CAD build for the part. Positions are in the model's coordinates, mm. Face numbers are marked on the shaded views. Coordinates: 2 decimals unless noted, no trailing zeros. Order: outer loops, then holes, each group sorted by start corner. A loop starts at its lowest first (then second) coordinate and runs counter-clockwise, first axis right, second up. Notation, with made-up numbers: M 68.25,13 L 83.25,13 A21 ccw 83.25,51 Z; hole C -16,38 d11. An arc over 180 degrees is marked long. One line per item, written item: value.
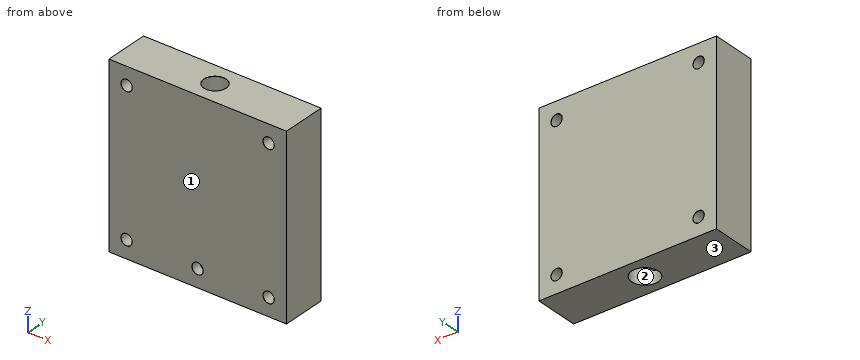
from build123d import *

# Parameters (mm, degrees)
ESQUISSE1_W                                         = 40
ESQUISSE1_H                                         = 40
BOSS_EXTRU_1_DEPTH                                  = 10
DIAM_TRE_DU_PER_AGE_4_0_4_1_D                       = 4
TROU_POUR_TARAUDAGE_POUR_TROU_TARAUD_M6_D           = 5
TROU_POUR_TARAUDAGE_POUR_TROU_TARAUD_M6_DEPTH       = 8
TROU_POUR_TARAUDAGE_POUR_TROU_TARAUD_M6_CSINK_D     = 5.05
TROU_POUR_TARAUDAGE_POUR_TROU_TARAUD_M6_CSINK_ANGLE = 90
TROU_POUR_TARAUDAGE_POUR_TROU_TARAUD_M6_TIP         = 1.502151548
DIAM_TRE_DU_PER_AGE_6_0_6_1_D                       = 6
DIAM_TRE_DU_PER_AGE_6_0_6_1_DEPTH                   = 20
DIAM_TRE_DU_PER_AGE_6_0_6_1_TIP                     = 1.802581857
TROU_POUR_TARAUDAGE_POUR_TROU_TARAUD_2_COUNT        = 2
TROU_POUR_TARAUDAGE_POUR_TROU_TARAUD_2_PITCH        = 32
TROU_POUR_TARAUDAGE_POUR_TROU_TARAUD_3_COUNT        = 2
TROU_POUR_TARAUDAGE_POUR_TROU_TARAUD_3_PITCH        = 45.254833996
TROU_POUR_TARAUDAGE_POUR_TROU_TARAUD_4_COUNT        = 2
TROU_POUR_TARAUDAGE_POUR_TROU_TARAUD_4_PITCH        = 32
TROU_POUR_TARAUDAGE_POUR_TROU_TARAUD_5_D            = 2.5
TROU_POUR_TARAUDAGE_POUR_TROU_TARAUD_5_DEPTH        = 5
TROU_POUR_TARAUDAGE_POUR_TROU_TARAUD_5_CSINK_D      = 2.55
TROU_POUR_TARAUDAGE_POUR_TROU_TARAUD_5_CSINK_ANGLE  = 90
TROU_POUR_TARAUDAGE_POUR_TROU_TARAUD_5_TIP          = 0.751075774


with BuildPart() as part:
    # Esquisse1 → Boss.-Extru.1 (new body)
    with BuildSketch(Plane(origin=(0, 0, 0), x_dir=(1, 0, 0), z_dir=(0, 1, 0))):
        with Locations((20, 20)):
            Rectangle(ESQUISSE1_W, ESQUISSE1_H)
    extrude(amount=BOSS_EXTRU_1_DEPTH)

    # Diamètre du perçage Ø4.0 (4)1 (through all)
    with Locations(Plane.XY):
        with Locations((20, 5)):
            Hole(DIAM_TRE_DU_PER_AGE_4_0_4_1_D / 2)

    # Trou pour taraudage pour trou taraudé M61
    with Locations(Plane.XY):
        with Locations((20, 5)):
            CounterSinkHole(TROU_POUR_TARAUDAGE_POUR_TROU_TARAUD_M6_D / 2, TROU_POUR_TARAUDAGE_POUR_TROU_TARAUD_M6_CSINK_D / 2, depth=TROU_POUR_TARAUDAGE_POUR_TROU_TARAUD_M6_DEPTH, counter_sink_angle=TROU_POUR_TARAUDAGE_POUR_TROU_TARAUD_M6_CSINK_ANGLE)
            with Locations((0, 0, -(TROU_POUR_TARAUDAGE_POUR_TROU_TARAUD_M6_DEPTH + TROU_POUR_TARAUDAGE_POUR_TROU_TARAUD_M6_TIP / 2))):  # 118° drill point
                Cone(0, TROU_POUR_TARAUDAGE_POUR_TROU_TARAUD_M6_D / 2, TROU_POUR_TARAUDAGE_POUR_TROU_TARAUD_M6_TIP, mode=Mode.SUBTRACT)

    # Diamètre du perçage Ø6.0 (6)1
    with Locations(Plane(origin=(0, 0, -40), x_dir=(-1, 0, 0), z_dir=(0, 0, -1))):
        with Locations((-20, 5)):
            Hole(DIAM_TRE_DU_PER_AGE_6_0_6_1_D / 2, depth=DIAM_TRE_DU_PER_AGE_6_0_6_1_DEPTH)
            with Locations((0, 0, -(DIAM_TRE_DU_PER_AGE_6_0_6_1_DEPTH + DIAM_TRE_DU_PER_AGE_6_0_6_1_TIP / 2))):  # 118° drill point
                Cone(0, DIAM_TRE_DU_PER_AGE_6_0_6_1_D / 2, DIAM_TRE_DU_PER_AGE_6_0_6_1_TIP, mode=Mode.SUBTRACT)

    # Esquisse17 → Trou pour taraudage pour trou taraud_ M3 (revolve, cut)
    with BuildSketch(Plane(origin=(4, 0, -4), x_dir=(0, 0, -1), z_dir=(1, 0, 0))):
        Polygon((0, 0), (0, 10), (1.275, 10), (1.25, 9.975), (1.25, 0.025), (1.275, 0), align=None)
    trou_pour_taraudage_pour_trou_taraud_m3 = revolve(axis=Axis((4, -6.35, -4), (0, 1, 0)), mode=Mode.SUBTRACT)

    # Trou pour taraudage pour trou taraud 2: Trou pour taraudage pour trou taraud_ M3 ×2
    with Locations(*[(i * TROU_POUR_TARAUDAGE_POUR_TROU_TARAUD_2_PITCH, 0, 0) for i in range(1, TROU_POUR_TARAUDAGE_POUR_TROU_TARAUD_2_COUNT)]):
        add(trou_pour_taraudage_pour_trou_taraud_m3, mode=Mode.SUBTRACT)

    # Trou pour taraudage pour trou taraud 3: Trou pour taraudage pour trou taraud_ M3 ×2
    with Locations(*[Vector(0.7071067811865475, 0, -0.7071067811865476) * (i * TROU_POUR_TARAUDAGE_POUR_TROU_TARAUD_3_PITCH) for i in range(1, TROU_POUR_TARAUDAGE_POUR_TROU_TARAUD_3_COUNT)]):
        add(trou_pour_taraudage_pour_trou_taraud_m3, mode=Mode.SUBTRACT)

    # Trou pour taraudage pour trou taraud 4: Trou pour taraudage pour trou taraud_ M3 ×2
    with Locations(*[(0, 0, -i * TROU_POUR_TARAUDAGE_POUR_TROU_TARAUD_4_PITCH) for i in range(1, TROU_POUR_TARAUDAGE_POUR_TROU_TARAUD_4_COUNT)]):
        add(trou_pour_taraudage_pour_trou_taraud_m3, mode=Mode.SUBTRACT)

    # Trou pour taraudage pour trou taraud 5
    with Locations(Plane(origin=(0, 0, 0), x_dir=(-1, 0, 0), z_dir=(0, -1, 0))):
        with Locations((-20, 36)):
            CounterSinkHole(TROU_POUR_TARAUDAGE_POUR_TROU_TARAUD_5_D / 2, TROU_POUR_TARAUDAGE_POUR_TROU_TARAUD_5_CSINK_D / 2, depth=TROU_POUR_TARAUDAGE_POUR_TROU_TARAUD_5_DEPTH, counter_sink_angle=TROU_POUR_TARAUDAGE_POUR_TROU_TARAUD_5_CSINK_ANGLE)
            with Locations((0, 0, -(TROU_POUR_TARAUDAGE_POUR_TROU_TARAUD_5_DEPTH + TROU_POUR_TARAUDAGE_POUR_TROU_TARAUD_5_TIP / 2))):  # 118° drill point
                Cone(0, TROU_POUR_TARAUDAGE_POUR_TROU_TARAUD_5_D / 2, TROU_POUR_TARAUDAGE_POUR_TROU_TARAUD_5_TIP, mode=Mode.SUBTRACT)


solid = part.part
Q1. Slice it at A-A (z = -36). List the corners of the cut face in (x, y) (3 decimals).
Recorded:
outline: M 0,0 L 2.725,0 L 2.75,0.025 L 2.75,9.975 L 2.725,10 L 0,10 Z; M 5.25,0.025 L 5.275,0 L 18.725,0 L 18.75,0.025 L 18.75,2.273 A3 cw long 21.25,2.273 L 21.25,0.025 L 21.275,0 L 34.725,0 L 34.75,0.025 L 34.75,9.975 L 34.725,10 L 5.275,10 L 5.25,9.975 Z; M 37.25,0.025 L 37.275,0 L 40,0 L 40,10 L 37.275,10 L 37.25,9.975 Z
Q2. Slice it at C-C (z = -10.5). List the corners of the cut face in (x, y).
Recorded:
outline: M 0,0 L 40,0 L 40,10 L 0,10 Z; hole C 20,5 d4
Q3. Slice it at B-B (x = 4). List the corners of the cut face in (y, z) (3 decimals).
Recorded:
outline: M 0,-40 L 10,-40 L 10,-37.275 L 9.975,-37.25 L 0.025,-37.25 L 0,-37.275 Z; M 0,-34.725 L 0.025,-34.75 L 9.975,-34.75 L 10,-34.725 L 10,-5.275 L 9.975,-5.25 L 0.025,-5.25 L 0,-5.275 Z; M 0,-2.725 L 0.025,-2.75 L 9.975,-2.75 L 10,-2.725 L 10,0 L 0,0 Z
Q4. Mould opens along Y. For the marked faces 1, 2 and 3 say: released by +Y, released by -Y, zero draft, split by the parting line, or undercut.
Recorded:
face 1: released by -Y
face 2: undercut
face 3: zero draft
Q5. Slice it at D-D (y = 6.5). Give the number of separate pieces and of enclosed holes in the cut face, plus the area to 3 significant figures.
Recorded:
separate pieces: 2
enclosed holes: 4
area: 1,410 mm^2
Q6. Drill centre lines: line 1 along Z through (x, y) = (4, 3.75); line 2 along X through (y, z) = (2, -4); line 3 along X through (y, z) = (1, -36). Where is each one in solid material? Low to high.
Recorded:
line 1: z = -40 to -37.25, -34.75 to -5.25, -2.75 to 0
line 2: x = 0 to 2.75, 5.25 to 34.75, 37.25 to 40
line 3: x = 0 to 2.75, 5.25 to 18.75, 21.25 to 34.75, 37.25 to 40
Q7. Pin check, flat tips, straight feed: pin 1 Ø1.5 at (x, z) = (20, -36) entering from -Y; pin 2 Ø3.5 at (x, y) = (20, 5) entering from -Z. Stop position of each tip, or through.
Recorded:
pin 1: stops at y = 7.9
pin 2: passes through
